Here's how the part is built. I have some questions about the finished solid (model axes, mm). Face numbers are marked on the shaded views. A direction names the side the tool comes from. Coordinates: 2 decimals unless noted, no trailing zeros. Order: outer loops, then holes, each group sorted by start corner. A loop starts at its lowest first (then second) coordinate and runs counter-clockwise, first axis right, second up. Notation, with made-up numbers: (4.5, 71) -> (61.5, 71) arc R6 ccw to (61.5, 76) -> close; hole circle Ø10 at (0.5, -5.5). An arc over 180 degrees is marked (long way). One line per item, written item: value. Start each with the question number.
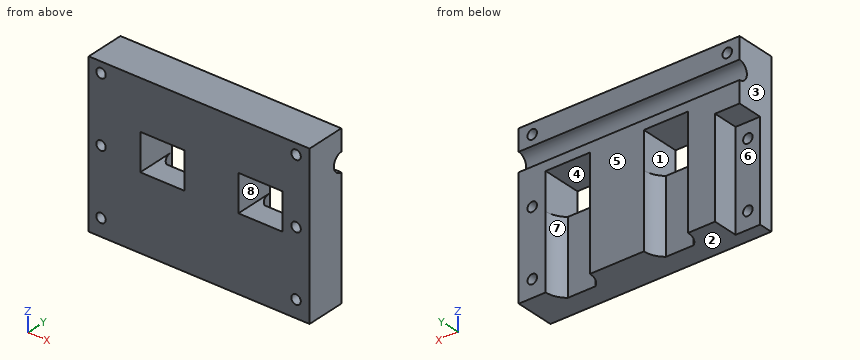
```python
from build123d import *

# Parameters (mm, degrees)
BOSS_EXTRUDE1_DEPTH  = 38.1
SKETCH7_W            = 101.6
SKETCH7_H            = 20.32
BOSS_EXTRUDE2_DEPTH  = 44.45
BOSS_EXTRUDE9_DEPTH  = 12.7
SKETCH8_W            = 22.86
SKETCH8_H            = 19.05
CUT_EXTRUDE1_DEPTH   = 20.32
CUT_EXTRUDE2_START   = -101.6
SKETCH9_R            = 4.826
CUT_EXTRUDE2_DEPTH   = 114.3
LPATTERN1_COUNT      = 3
LPATTERN1_PITCH      = 34.067332164
LPATTERN1_COUNT_DIR2 = 2
LPATTERN1_PITCH_DIR2 = 100.965


with BuildPart() as part:
    # Sketch1 → Boss-Extrude1 (new body)
    with BuildSketch(Plane.XY):
        with BuildLine():
            Line((-50.8, 0), (50.8, 0))
            Line((50.8, 0), (50.8, 20.32))
            Line((50.8, 20.32), (36.83, 20.32))
            ThreePointArc((36.83, 20.32), (35.714076836, 15.394076836), (32.584204897, 11.43))
            Line((32.584204897, 11.43), (18.215795103, 11.43))
            ThreePointArc((18.215795103, 11.43), (15.085923164, 15.394076836), (13.97, 20.32))
            Line((13.97, 20.32), (-13.97, 20.32))
            ThreePointArc((-13.97, 20.32), (-15.085923164, 15.394076836), (-18.215795103, 11.43))
            Line((-18.215795103, 11.43), (-32.584204897, 11.43))
            ThreePointArc((-32.584204897, 11.43), (-35.714076836, 15.394076836), (-36.83, 20.32))
            Line((-36.83, 20.32), (-50.8, 20.32))
            Line((-50.8, 20.32), (-50.8, 0))
        make_face()
    extrude(amount=BOSS_EXTRUDE1_DEPTH)

    # Sketch7 → Boss-Extrude2 (add)
    with BuildSketch(Plane.XY.offset(38.1)):
        with Locations((0, 10.16)):
            Rectangle(SKETCH7_W, SKETCH7_H)
    extrude(amount=BOSS_EXTRUDE2_DEPTH)

    # Sketch21 → Boss-Extrude9 (add)
    with BuildSketch(Plane.ZY.offset(50.8)):
        Polygon((0, 7.112), (0, 0), (68.41445042, 0), (82.55, 0), (82.55, 7.153488119), (82.55, 20.32), (50.8, 20.32), (50.8, 7.112), align=None)
    extrude(amount=BOSS_EXTRUDE9_DEPTH)

    # Sketch8 → Cut-Extrude1 (cut)
    with BuildSketch(Plane(origin=(0, 20.32, 0), x_dir=(1, 0, 0), z_dir=(0, 1, 0))):
        with Locations((-25.4, -47.625)):
            Rectangle(SKETCH8_W, SKETCH8_H)
        with Locations((25.4, -47.625)):
            Rectangle(SKETCH8_W, SKETCH8_H)
    extrude(amount=-CUT_EXTRUDE1_DEPTH, mode=Mode.SUBTRACT)

    # Sketch5 → #10 (0.1935) Diameter Hole1 (revolve, cut)
    with BuildSketch(Plane(origin=(-57.15, 20.32, 8.89), x_dir=(0, 0, 1), z_dir=(1, 0, 0))):
        Polygon((0, 0), (0, 25.4), (2.45745, 23.923415072), (2.45745, 0), align=None)
    f_10_0_1935_diameter_hole1 = revolve(axis=Axis((-57.15, 26.67, 8.89), (0, -1, 0)), mode=Mode.SUBTRACT)

    # Sketch9 → Cut-Extrude2 (cut)
    with BuildSketch(Plane.ZY.offset(50.8).offset(CUT_EXTRUDE2_START)):
        with Locations((66.675, 20.447)):
            Circle(SKETCH9_R)
    extrude(amount=CUT_EXTRUDE2_DEPTH, mode=Mode.SUBTRACT)

    # LPattern1: 10 _0.1935_ Diameter Hole1 3 × 2
    with Locations(*[(j * LPATTERN1_PITCH_DIR2, 0, i * LPATTERN1_PITCH) for i in range(LPATTERN1_COUNT) for j in range(LPATTERN1_COUNT_DIR2) if (i, j) != (0, 0)]):
        add(f_10_0_1935_diameter_hole1, mode=Mode.SUBTRACT)


solid = part.part
```
Q1. Imagine slicing it at A-A (z = 8.89). Write out the boundary of the cut face in (x, y), plus the area to 3 significant figures.
Q2. For the marked faces 5, 6, 7 and 8, which set-ups out of +Z, -Z, +X, -X, +Y, -Y let a thin tool reach every point of the face, with its end or its side?
Q3. If we mould it in two halves opening along X, with no side actions, what happens to the marked faces 1, 2, 3 and 4? For each: +X half, -X half, draft (parallel to the pull), parting line (faces both ways), or undercut.
Q4. I need wall thicknesses on line 1 (X direction, y = 7.5, z = 52); line 2 (X direction, y = 7.75, z = 44); line 3 (X direction, y = 2.5, z = 9.5). Which ranges of each line are inside material? Lowest first, please.
Q5. Imagine slicing it at D-D (z = 43). Write out the boundary of the cut face in (x, y).
Q6. For P1, Ø4.5, axis at x = 22, z = 17, coming from the +Y side; P2, Ø6.5, axis at x = -59, y = 17, coming from the -Z side; P3, Ø4, axis at x = 23.5, y = 16, coming from the -Z side, each with a flat end and sliding along its axis, tell me the tip position at first contact or that it passes through.
Q7. Imagine slicing it at C-C (y = 18.75). Count the separate pieces of the cut face and the enclosed holes in it, plus the area to 3 significant figures.
Q8. Imagine slicing it at B-B (x = 21). Write out the boundary of the cut face in (y, z) (3 decimals).
Completed:
1. outline: (-63.5, 0) -> (-59.61, 0) -> (-59.61, 7.11) -> (-63.5, 7.11) -> close; (-54.69, 0) -> (41.36, 0) -> (41.36, 20.32) -> (36.83, 20.32) arc R11.43 cw to (32.58, 11.43) -> (18.22, 11.43) arc R11.43 cw to (13.97, 20.32) -> (-13.97, 20.32) arc R11.43 cw to (-18.22, 11.43) -> (-32.58, 11.43) arc R11.43 cw to (-36.83, 20.32) -> (-50.8, 20.32) -> (-50.8, 7.11) -> (-54.69, 7.11) -> close; (46.27, 0) -> (50.8, 0) -> (50.8, 20.32) -> (46.27, 20.32) -> close
1. area: 1,660 mm2
2. face 5: +Z, -Z, +X, -X, +Y
2. face 6: -Z, -X, +Y
2. face 7: -Z, +Y
2. face 8: +Y, -Y
3. face 1: undercut
3. face 2: draft
3. face 3: -X half
3. face 4: undercut
4. line 1: x = -63.5 to -36.83, -13.97 to 13.97, 36.83 to 50.8
4. line 2: x = -50.8 to -36.83, -13.97 to 13.97, 36.83 to 41.59, 46.04 to 50.8
4. line 3: x = -63.5 to -59.53, -54.77 to 41.43, 46.2 to 50.8
5. outline: (-63.5, 0) -> (-59.61, 0) -> (-59.61, 7.11) -> (-63.5, 7.11) -> close; (-54.69, 0) -> (-36.83, 0) -> (-36.83, 20.32) -> (-50.8, 20.32) -> (-50.8, 7.11) -> (-54.69, 7.11) -> close; (-13.97, 0) -> (13.97, 0) -> (13.97, 20.32) -> (-13.97, 20.32) -> close; (36.83, 0) -> (41.36, 0) -> (41.36, 20.32) -> (36.83, 20.32) -> close; (46.27, 0) -> (50.8, 0) -> (50.8, 20.32) -> (46.27, 20.32) -> close
6. P1: stops at y = 11.43
6. P2: stops at z = 50.8
6. P3: stops at z = 57.15
7. separate pieces: 2
7. enclosed holes: 4
7. area: 5,090 mm2
8. outline: (0, 0) -> (11.43, 0) -> (11.43, 38.1) -> (0, 38.1) -> close; (0, 57.15) -> (20.32, 57.15) -> (20.32, 61.851) arc R4.826 cw to (20.32, 71.499) -> (20.32, 82.55) -> (0, 82.55) -> close
